Check sheet for the modelled part. Datum: model origin and axes. Units: mm. Face numbers are marked on the shaded views. A direction names the side the tool comes from. Coordinates: 2 decimals unless noted, no trailing zeros. Loops run counter-clockwise (first coordinate to the right, second up) from the corner with the lowest first, then second, coordinate; pieces in that order, holes last. Notation, with made-up numbers: (50, -28) -> (89, -28) arc R18 cw to (89, -21) -> close; hole circle Ø2 at (-20, 10.25). An arc over 180 degrees is marked (long way). Use one line per item in the form item = value.
from build123d import *

# Parameters (mm, degrees)
F0_W     = 76.2
F0_H     = 25.4
F0_R     = 1.5875
F1_DEPTH = 25.4
F2_R     = 2.54
F3_DEPTH = 7.62
F4_W     = 25.4
F4_H     = 12.7
F5_DEPTH = 6.35
F6_W     = 6.35
F6_H     = 3.175
F7_DEPTH = 12.7
F8_DEPTH = 19.05


with BuildPart() as f1:
    # F0 (on Front) → F1 (new body)
    with BuildSketch(Plane.XZ):
        Rectangle(F0_W, F0_H)
        with Locations((-4.7625, 0)):
            Circle(F0_R, mode=Mode.SUBTRACT)
        with Locations((4.7625, 0)):
            Circle(F0_R, mode=Mode.SUBTRACT)
        with Locations((-4.7625, 0)):
            Circle(F0_R)
        with Locations((4.7625, 0)):
            Circle(F0_R)
    extrude(amount=-F1_DEPTH)

    # F2 (on face) → F3 (join)
    with BuildSketch(Plane(origin=(0, 25.4, 0), x_dir=(-1, 0, 0), z_dir=(0, 1, 0))):
        Circle(F2_R)
    extrude(amount=F3_DEPTH)

    # F4 (on face) → F5 (join)
    with BuildSketch(Plane(origin=(0, 33.02, 0), x_dir=(-1, 0, 0), z_dir=(0, 1, 0))):
        Rectangle(F4_W, F4_H)
    extrude(amount=F5_DEPTH)

    # F6 (on face) → F7 (join)
    with BuildSketch(Plane(origin=(0, 39.37, 0), x_dir=(-1, 0, 0), z_dir=(0, 1, 0))):
        with Locations((9.525, 0)):
            Rectangle(F6_W, F6_H)
    extrude(amount=F7_DEPTH)

    # F0 (on Front) → F8 (cut)
    with BuildSketch(Plane.XZ):
        with Locations((-4.7625, 0)):
            Circle(F0_R)
        with Locations((4.7625, 0)):
            Circle(F0_R)
    extrude(amount=-F8_DEPTH, mode=Mode.SUBTRACT)


solid = f1.part
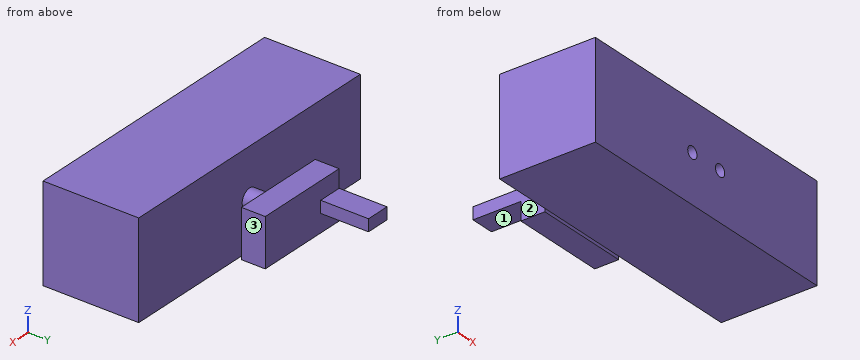
(1) Section check D-D, the plane x = 15.5. Record the boundary of the cut face in (y, z).
Established:
outline = (0, -12.7) -> (25.4, -12.7) -> (25.4, 12.7) -> (0, 12.7) -> close
(2) Tool access check on the marked faces 1, 2 and 3. Record the directions out of +Z, -Z, +X, -X, +Y, -Y that give a thin tool (end or side, any length) a straight path to the whole face; none if there is none.
Established:
face_1 = -Z, +X, -X, +Y
face_2 = +Z, -Z, -X, +Y
face_3 = +Z, -Z, +X, +Y
(3) Scan lines: line 1 along Y through (x, z) = (8, 5.5); line 2 along Y through (x, z) = (-18.5, -6.25); line 3 along Y through (x, z) = (-8.5, 0.5). Record each from-to range of solid material in increasing order.
Established:
line_1 = 0 to 25.4, 33.02 to 39.37
line_2 = 0 to 25.4
line_3 = 0 to 25.4, 33.02 to 52.07
(4) Section check B-B, the plane x = 0. Record the boundary of the cut face in (y, z), plus the area to 3 significant figures.
Established:
outline = (0, -12.7) -> (25.4, -12.7) -> (25.4, -2.54) -> (33.02, -2.54) -> (33.02, -6.35) -> (39.37, -6.35) -> (39.37, 6.35) -> (33.02, 6.35) -> (33.02, 2.54) -> (25.4, 2.54) -> (25.4, 12.7) -> (0, 12.7) -> close
area = 765 mm²
(5) Section check A-A, the plane z = 0. Record the boundary of the cut face in (x, y) (3 decimals), plus the area to 3 significant figures.
Established:
outline = (-38.1, 0) -> (-6.35, 0) -> (-6.35, 19.05) -> (-3.175, 19.05) -> (-3.175, 0) -> (3.175, 0) -> (3.175, 19.05) -> (6.35, 19.05) -> (6.35, 0) -> (38.1, 0) -> (38.1, 25.4) -> (2.54, 25.4) -> (2.54, 33.02) -> (12.7, 33.02) -> (12.7, 39.37) -> (-6.35, 39.37) -> (-6.35, 52.07) -> (-12.7, 52.07) -> (-12.7, 33.02) -> (-2.54, 33.02) -> (-2.54, 25.4) -> (-38.1, 25.4) -> close
area = 2,100 mm²
(6) Go/stop test with flat-tipped pins: P1, Ø7, axis at x = 3.5, y = 35.5, coming from the -Z side; P2, Ø4, axis at y = 47, z = 2.5, coming from the -X side; P3, Ø5, axis at y = 35.5, z = -0.5, coming from the +X side; P4, Ø6.5, axis at x = 3.5, z = -1, coming from the -Y side. Record where each tip stops, or that it passes through.
Established:
P1 = -6.35
P2 = -12.7
P3 = 12.7
P4 = 0
(7) Section check C-C, the plane y = 29. Record the boundary of the cut face in (x, z), plus the area to 3 significant figures.
Established:
outline = circle Ø5.08 at (0, 0)
area = 20.3 mm²
